Could you check a few things on this drawing? It's one solid part, dimensions in mm from its lowest x, y, z. A direction names the side the tool comes from. Give positions to 0.01 mm unless a question says otherwise; leave off trailing zeros. Order: outer loops, then holes, each group sorted by start corner. A loop starts at its lowest first (then second) coordinate and runs counter-clockwise, first axis right, second up.
(1) If we mould it in two halves opening along X, with no side actions, what happens to the marked faces 5, 6 and 7? For each: released by +X, released by -X, zero draft, split by the parting line, or undercut.
(2) Imagine slicing it at A-A, the plane y = 27. Write out the boundary of the cut face in (x, z).
(3) On a 3-axis mill with a long thin cutter (end or side, diameter ignored), from which of +Z, -Z, +X, -X, +Y, -Y can I reach the whole of each face in a straight line? I mean the marked faces 1, 2, 3 and 4. Say none if no direction works.
(4) Imagine slicing it at C-C, the plane x = 6.5. Write out the boundary of the cut face in (y, z).
(5) If I drill on probe 1 along Z at (x, y) = (3, 3); probe 2 along X at (y, z) = (25, 7.5); probe 3 along Z at (x, y) = (7.3, 27), over which ranges is the centre line in solid material (lowest first)?
(6) Will these pins go through, and if not, where does the flat tip stop? pin 1 (2 mm diameter, centred on y = 27, z = 2.5, fed in from +X); pin 2 (1.5 mm diameter, centred on x = 5, y = 12, fed in from -Z); pin 3 (3 mm diameter, centred on x = 1.5, y = 8.5, fed in from +Z); pin 4 (4 mm diameter, centred on x = 7, z = 3, fed in from -Y).
(7) Imagine slicing it at B-B, the plane z = 20.25. Write out the boundary of the cut face in (x, y).
(8) Imagine slicing it at D-D, the plane z = 2.5. Write out the boundary of the cut face in (x, y), then the cut area to 3 significant figures.
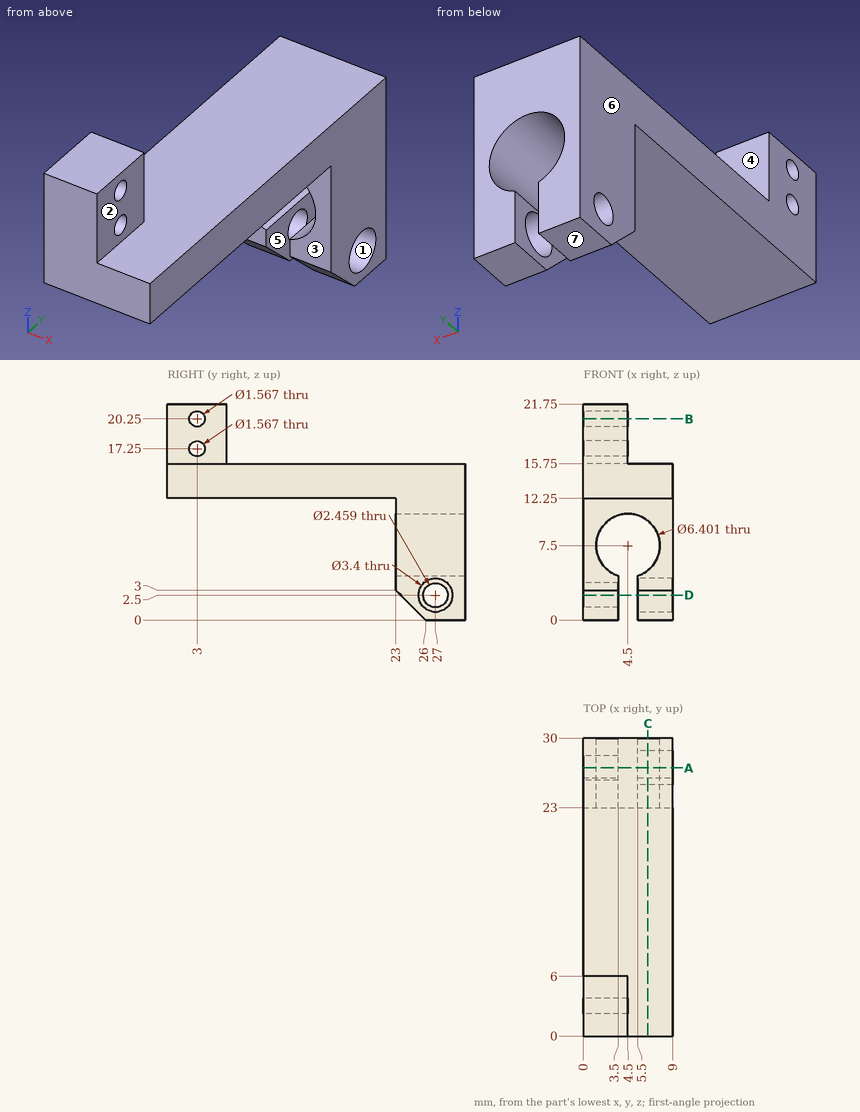
Answer block:
1. face 5: undercut
1. face 6: released by -X
1. face 7: zero draft
2. outline: (0, 0) - (3.5, 0) - (3.5, 1.27) - (0, 1.27) - close; (0, 3.73) - (3.5, 3.73) - (3.5, 4.46) arc R3.2 cw (long way) to (5.5, 4.46) - (5.5, 4.2) - (9, 4.2) - (9, 15.75) - (0, 15.75) - close; (5.5, 0) - (9, 0) - (9, 0.8) - (5.5, 0.8) - close
3. face 1: +X
3. face 2: +Z, +X, +Y, -Y
3. face 3: -Z, +X, -X, -Y
3. face 4: +Z, +X, -X, +Y
4. outline: (0, 12.25) - (23, 12.25) - (23, 10) - (30, 10) - (30, 15.75) - (0, 15.75) - close; (23, 3) - (26, 0) - (30, 0) - (30, 5) - (23, 5) - close; hole circle Ø3.4 at (27, 2.5)
5. probe 1: z = 12.25 to 16.47, 18.03 to 19.47, 21.03 to 21.75
5. probe 2: x = 0 to 1.3, 7.7 to 9
5. probe 3: z = 0 to 0.8, 4.2 to 5.95, 9.05 to 15.75
6. pin 1: passes through
6. pin 2: stops at z = 12.25
6. pin 3: stops at z = 15.75
6. pin 4: stops at y = 23
7. outline: (0, 0) - (4.5, 0) - (4.5, 2.22) - (0, 2.22) - close; (0, 3.78) - (4.5, 3.78) - (4.5, 6) - (0, 6) - close
8. outline: (0, 23.5) - (3.5, 23.5) - (3.5, 25.77) - (0, 25.77) - close; (0, 28.23) - (3.5, 28.23) - (3.5, 30) - (0, 30) - close; (5.5, 23.5) - (9, 23.5) - (9, 25.3) - (5.5, 25.3) - close; (5.5, 28.7) - (9, 28.7) - (9, 30) - (5.5, 30) - close
8. area: 25.0 mm2
